Source: CAD feature listing. Evaluate the final solid. Frame: model axes, mm. A direction names the side the tool comes from. Coordinates: 2 decimals unless noted, no trailing zeros. Order: outer loops, then holes, each group sorted by start corner. A loop starts at its lowest first (then second) coordinate and runs counter-clockwise, first axis right, second up.
```python
from build123d import *

# Parameters (mm, degrees)
F0_W      = 8
F0_H      = 2.5
F1_DEPTH  = 16.25
F3_DEPTH  = 16.2
F5_W      = 1.2
F5_H      = 18
F7_DEPTH  = 3.3507126627
F8_DEPTH  = 5.5
F10_DEPTH = 0.1
F12_DEPTH = 0.1


with BuildPart() as f1:
    # F0 (on Top) → F1 (new body)
    with BuildSketch(Plane.XY):
        with BuildLine():
            Line((-3.475, -2.275), (3.475, -2.275))
            ThreePointArc((3.475, -2.275), (5.0659902577, -1.6159902577), (5.725, -0.025))
            Line((5.725, -0.025), (5.725, 0.025))
            ThreePointArc((5.725, 0.025), (5.0659902577, 1.6159902577), (3.475, 2.275))
            Line((3.475, 2.275), (-3.475, 2.275))
            ThreePointArc((-3.475, 2.275), (-5.0659902577, 1.6159902577), (-5.725, 0.025))
            Line((-5.725, 0.025), (-5.725, -0.025))
            ThreePointArc((-5.725, -0.025), (-5.0659902577, -1.6159902577), (-3.475, -2.275))
        make_face()
        Rectangle(F0_W, F0_H, mode=Mode.SUBTRACT)
        Rectangle(F0_W, F0_H)
    extrude(amount=F1_DEPTH)


with BuildPart() as f3:
    # F2 (on Top) → F3 (new body)
    with BuildSketch(Plane.XY):
        with BuildLine():
            Line((-7, -4), (7, -4))
            ThreePointArc((7, -4), (8.4142135624, -3.4142135624), (9, -2))
            Line((9, -2), (9, 2))
            ThreePointArc((9, 2), (8.4142135624, 3.4142135624), (7, 4))
            Line((7, 4), (-7, 4))
            Line((-7, 4), (-7, -4))
        make_face()
        with BuildLine():
            ThreePointArc((-9, -2), (-8.9681207868, -2.3556691844), (-8.8734994313, -2.6999999151))
            Line((-8.8734994313, -2.6999999151), (-7.9164700583, -2.6999999151))
            Line((-7.9164700583, -2.6999999151), (-7.9164700583, 2.6999999151))
            Line((-7.9164700583, 2.6999999151), (-8.8734994313, 2.6999999151))
            ThreePointArc((-8.8734994313, 2.6999999151), (-8.9681207868, 2.3556691844), (-9, 2))
            Line((-9, 2), (-9, -2))
        make_face()
        with BuildLine():
            ThreePointArc((-8.8734994313, -2.6999999151), (-8.1401754623, -3.6431676467), (-7, -4))
            Line((-7, -4), (-7, 4))
            ThreePointArc((-7, 4), (-8.1401754623, 3.6431676467), (-8.8734994313, 2.6999999151))
            Line((-8.8734994313, 2.6999999151), (-7.9164700583, 2.6999999151))
            Line((-7.9164700583, 2.6999999151), (-7.9164700583, -2.6999999151))
            Line((-7.9164700583, -2.6999999151), (-8.8734994313, -2.6999999151))
        make_face()
    extrude(amount=F3_DEPTH)

    # F6: cut F1
    add(f1.part, mode=Mode.SUBTRACT)

    # F5 (on face) → F7 (cut, through all)
    with BuildSketch(Plane.YZ.offset(9)):
        with Locations((0, 8)):
            Rectangle(F5_W, F5_H)
    extrude(amount=-F7_DEPTH, mode=Mode.SUBTRACT)

    # F2 (on Top) → F8 (join)
    with BuildSketch(Plane.XY):
        with BuildLine():
            Line((-10.7359819859, -4), (-7, -4))
            ThreePointArc((-7, -4), (-8.1401754623, -3.6431676467), (-8.8734994313, -2.6999999151))
            Line((-8.8734994313, -2.6999999151), (-10.7359819859, -2.6999999151))
            ThreePointArc((-10.7359819859, -2.6999999151), (-11.9380634539, -2.202081468), (-12.435981901, -1))
            Line((-12.435981901, -1), (-12.435981901, 1))
            ThreePointArc((-12.435981901, 1), (-11.9380634539, 2.202081468), (-10.7359819859, 2.6999999151))
            Line((-10.7359819859, 2.6999999151), (-8.8734994313, 2.6999999151))
            ThreePointArc((-8.8734994313, 2.6999999151), (-8.1401754623, 3.6431676467), (-7, 4))
            Line((-7, 4), (-10.7359819859, 4))
            ThreePointArc((-10.7359819859, 4), (-12.8573023295, 3.1213203436), (-13.7359819859, 1))
            Line((-13.7359819859, 1), (-13.7359819859, -1))
            ThreePointArc((-13.7359819859, -1), (-12.8573023295, -3.1213203436), (-10.7359819859, -4))
        make_face()
    extrude(amount=F8_DEPTH)

    # F9 (on face) → F10 (join)
    with BuildSketch(Plane.XY.offset(16.2)):
        with BuildLine():
            Line((3.475, -2.0750000357), (-3.475, -2.0750000357))
            ThreePointArc((-3.475, -2.0750000357), (-4.9245689267, -1.4745689267), (-5.5250000357, -0.025))
            Line((-5.5250000357, -0.025), (-5.5250000357, 0.025))
            ThreePointArc((-5.5250000357, 0.025), (-4.9245689267, 1.4745689267), (-3.475, 2.0750000357))
            Line((-3.475, 2.0750000357), (3.475, 2.0750000357))
            ThreePointArc((3.475, 2.0750000357), (4.7156218246, 1.6569796674), (5.4502873731, 0.5733976115))
            Line((5.4502873731, 0.5733976115), (5.6502873373, 0.6))
            ThreePointArc((5.6502873373, 0.6), (4.8477253913, 1.8077296486), (3.475, 2.275))
            Line((3.475, 2.275), (-3.475, 2.275))
            ThreePointArc((-3.475, 2.275), (-5.0659902577, 1.6159902577), (-5.725, 0.025))
            Line((-5.725, 0.025), (-5.725, -0.025))
            ThreePointArc((-5.725, -0.025), (-5.0659902577, -1.6159902577), (-3.475, -2.275))
            Line((-3.475, -2.275), (3.475, -2.275))
            ThreePointArc((3.475, -2.275), (4.8477253913, -1.8077296486), (5.6502873373, -0.6))
            Line((5.6502873373, -0.6), (5.4502873731, -0.5733976115))
            ThreePointArc((5.4502873731, -0.5733976115), (4.7156218246, -1.6569796674), (3.475, -2.0750000357))
        make_face()
        with BuildLine():
            Line((9, -0.6), (5.6502873373, -0.6))
            ThreePointArc((5.6502873373, -0.6), (4.8477253913, -1.8077296486), (3.475, -2.275))
            Line((3.475, -2.275), (-3.475, -2.275))
            ThreePointArc((-3.475, -2.275), (-5.0659902577, -1.6159902577), (-5.725, -0.025))
            Line((-5.725, -0.025), (-5.725, 0.025))
            ThreePointArc((-5.725, 0.025), (-5.0659902577, 1.6159902577), (-3.475, 2.275))
            Line((-3.475, 2.275), (3.475, 2.275))
            ThreePointArc((3.475, 2.275), (4.8477253913, 1.8077296486), (5.6502873373, 0.6))
            Line((5.6502873373, 0.6), (9, 0.6))
            Line((9, 0.6), (9, 2))
            ThreePointArc((9, 2), (8.4142135624, 3.4142135624), (7, 4))
            Line((7, 4), (-7, 4))
            ThreePointArc((-7, 4), (-8.4142135624, 3.4142135624), (-9, 2))
            Line((-9, 2), (-9, -2))
            ThreePointArc((-9, -2), (-8.4142135624, -3.4142135624), (-7, -4))
            Line((-7, -4), (7, -4))
            ThreePointArc((7, -4), (8.4142135624, -3.4142135624), (9, -2))
            Line((9, -2), (9, -0.6))
        make_face()
    extrude(amount=F10_DEPTH)

    # F11 (on face) → F12 (join)
    with BuildSketch(Plane(origin=(0, 0, 0), x_dir=(1, 0, 0), z_dir=(0, 0, -1))):
        with BuildLine():
            ThreePointArc((5.4502873731, -0.5733976115), (4.7156218246, -1.6569796674), (3.475, -2.0750000357))
            Line((3.475, -2.0750000357), (-3.475, -2.0750000357))
            ThreePointArc((-3.475, -2.0750000357), (-4.9245689267, -1.4745689267), (-5.5250000357, -0.025))
            Line((-5.5250000357, -0.025), (-5.5250000357, 0.025))
            ThreePointArc((-5.5250000357, 0.025), (-4.9245689267, 1.4745689267), (-3.475, 2.0750000357))
            Line((-3.475, 2.0750000357), (3.475, 2.0750000357))
            ThreePointArc((3.475, 2.0750000357), (4.7156218246, 1.6569796674), (5.4502873731, 0.5733976115))
            Line((5.4502873731, 0.5733976115), (5.6502873373, 0.6))
            ThreePointArc((5.6502873373, 0.6), (4.8477253913, 1.8077296486), (3.475, 2.275))
            Line((3.475, 2.275), (-3.475, 2.275))
            ThreePointArc((-3.475, 2.275), (-5.0659902577, 1.6159902577), (-5.725, 0.025))
            Line((-5.725, 0.025), (-5.725, -0.025))
            ThreePointArc((-5.725, -0.025), (-5.0659902577, -1.6159902577), (-3.475, -2.275))
            Line((-3.475, -2.275), (3.475, -2.275))
            ThreePointArc((3.475, -2.275), (4.8477253913, -1.8077296486), (5.6502873373, -0.6))
            Line((5.6502873373, -0.6), (5.4502873731, -0.5733976115))
        make_face()
        with BuildLine():
            Line((9, -0.6), (5.6502873373, -0.6))
            ThreePointArc((5.6502873373, -0.6), (4.8477253913, -1.8077296486), (3.475, -2.275))
            Line((3.475, -2.275), (-3.475, -2.275))
            ThreePointArc((-3.475, -2.275), (-5.0659902577, -1.6159902577), (-5.725, -0.025))
            Line((-5.725, -0.025), (-5.725, 0.025))
            ThreePointArc((-5.725, 0.025), (-5.0659902577, 1.6159902577), (-3.475, 2.275))
            Line((-3.475, 2.275), (3.475, 2.275))
            ThreePointArc((3.475, 2.275), (4.8477253913, 1.8077296486), (5.6502873373, 0.6))
            Line((5.6502873373, 0.6), (9, 0.6))
            Line((9, 0.6), (9, 2))
            ThreePointArc((9, 2), (8.4142135624, 3.4142135624), (7, 4))
            Line((7, 4), (-7, 4))
            Line((-7, 4), (-10.7359819859, 4))
            ThreePointArc((-10.7359819859, 4), (-12.8573023295, 3.1213203436), (-13.7359819859, 1))
            Line((-13.7359819859, 1), (-13.7359819859, -1))
            ThreePointArc((-13.7359819859, -1), (-12.8573023295, -3.1213203436), (-10.7359819859, -4))
            Line((-10.7359819859, -4), (-7, -4))
            Line((-7, -4), (7, -4))
            ThreePointArc((7, -4), (8.4142135624, -3.4142135624), (9, -2))
            Line((9, -2), (9, -0.6))
        make_face()
        with BuildLine():
            Line((-10.7359819859, 2.6999999151), (-8.8734994313, 2.6999999151))
            ThreePointArc((-8.8734994313, 2.6999999151), (-8.9681207868, 2.3556691844), (-9, 2))
            Line((-9, 2), (-9, -2))
            ThreePointArc((-9, -2), (-8.9681207868, -2.3556691844), (-8.8734994313, -2.6999999151))
            Line((-8.8734994313, -2.6999999151), (-10.7359819859, -2.6999999151))
            ThreePointArc((-10.7359819859, -2.6999999151), (-11.9380634539, -2.202081468), (-12.435981901, -1))
            Line((-12.435981901, -1), (-12.435981901, 1))
            ThreePointArc((-12.435981901, 1), (-11.9380634539, 2.202081468), (-10.7359819859, 2.6999999151))
        make_face(mode=Mode.SUBTRACT)
    extrude(amount=F12_DEPTH)


solid = f3.part
```
1. Draft query along Z for faces 4 (the face through (-12.436, 0, 3)), 5 (the face through (-5.05, 1.63, 7.99)), 6 (the face through (-5.08, -1.6, 7.99)). Return one class per face: released by +Z, released by -Z, zero draft, split by the parting line, or undercut.
Findings:
face 4: zero draft
face 5: undercut
face 6: undercut
2. Ray query, line 1 (Y direction, x = 6, z = 4); line 2 (X direction, y = 2, z = 4.25); line 3 (Y direction, x = -1, z = 9.25) (3 decimals). Return the intervals inside material, ascending.
Findings:
line 1: y = -4 to -0.6, 0.6 to 4
line 2: x = -13.56 to -12.11, -9 to -4.55, 4.55 to 9
line 3: y = -4 to -2.275, 2.275 to 4
3. Section query D-D on z = 9.25. Return loops of the section in (x, y) (3 decimals), plus the area to 3 significant figures.
Findings:
outline: (-9, -2) arc R2 ccw to (-7, -4) - (7, -4) arc R2 ccw to (9, -2) - (9, -0.6) - (5.65, -0.6) arc R2.25 cw to (3.475, -2.275) - (-3.475, -2.275) arc R2.25 cw to (-5.725, -0.025) - (-5.725, 0.025) arc R2.25 cw to (-3.475, 2.275) - (3.475, 2.275) arc R2.25 cw to (5.65, 0.6) - (9, 0.6) - (9, 2) arc R2 ccw to (7, 4) - (-7, 4) arc R2 ccw to (-9, 2) - close
area: 88.9 mm2
4. Pin query (flat end, axial travel): P1, Ø3, axis at y = 1, z = 11, coming from the -X side. Return the tip coordinate at first contact, or that it passes through.
Findings:
P1: stops at x = -9
5. Section query C-C on y = 1.75. Return loops of the section in (x, z), plus the area to 3 significant figures.
Findings:
outline: (-13.64, -0.1) - (-12.26, -0.1) - (-12.26, 5.5) - (-13.64, 5.5) - close; (-9, -0.1) - (-4.58, -0.1) - (-4.58, 0) - (-4.92, 0) - (-4.92, 16.2) - (-4.58, 16.2) - (-4.58, 16.3) - (-9, 16.3) - close; (4.58, -0.1) - (9, -0.1) - (9, 16.3) - (4.58, 16.3) - (4.58, 16.2) - (4.92, 16.2) - (4.92, 0) - (4.58, 0) - close
area: 142 mm2
6. Section query A-A on x = 1. Return loops of the section in (y, z) (3 decimals).
Findings:
outline: (-4, -0.1) - (-2.075, -0.1) - (-2.075, 0) - (-2.275, 0) - (-2.275, 16.2) - (-2.075, 16.2) - (-2.075, 16.3) - (-4, 16.3) - close; (2.075, -0.1) - (4, -0.1) - (4, 16.3) - (2.075, 16.3) - (2.075, 16.2) - (2.275, 16.2) - (2.275, 0) - (2.075, 0) - close
7. Access query for faces 1 (the face through (4.86, 1.8, 7.99)), 2 (the face through (7, 0.6, 8)), 3 (the face through (-10, 2.7, 3)). Directions: +Z, -Z, +X, -X, +Y, -Y. A direction counts if a zero-diameter tool reaches every point of the face in a straight line with its end or side. Return the directions, or none.
Findings:
face 1: none
face 2: +Z, -Z, +X
face 3: +Z, -Z
